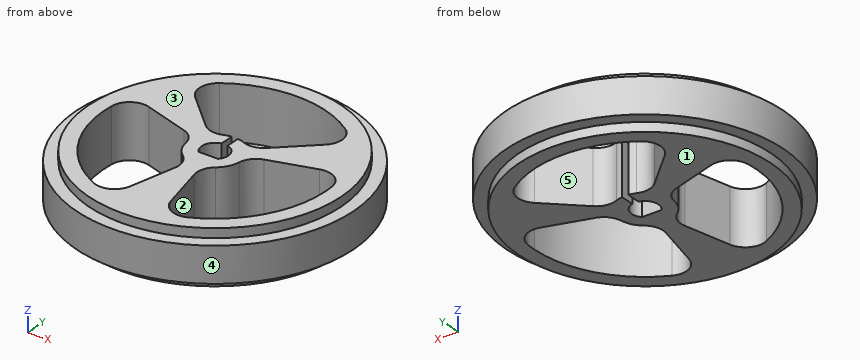
```python
from build123d import *

# Parameters (mm, degrees)
F3_DEPTH = 7
F4_R     = 2.5


with BuildPart() as f1:
    # F0 (on Front) → F1 (revolve)
    with BuildSketch(Plane.XZ):
        Polygon((-16.4, 0), (0, 0), (0, 7), (-16.4, 7), (-16.4, 5.8), (-18, 5.8), (-18, 1.2), (-16.4, 1.2), align=None)
    revolve(axis=Axis((0, 0, 3.5), (0, 0, -1)))

    # F2 (on Top) → F3 (cut, through all)
    with BuildSketch(Plane.XY):
        with BuildLine():
            Line((-0.4, 3.477068), (-0.4, 1.677982))
            ThreePointArc((-0.4, 1.677982), (-1.651125, 0.499411), (-1.262933, -1.175))
            Line((-1.262933, -1.175), (1.262933, -1.175))
            ThreePointArc((1.262933, -1.175), (1.651125, 0.499411), (0.4, 1.677982))
            Line((0.4, 1.677982), (0.4, 3.477068))
            ThreePointArc((0.4, 3.477068), (1.573642, 3.126284), (2.55453, 2.392567))
            Line((2.55453, 2.392567), (10.510067, 9.843703))
            ThreePointArc((10.510067, 9.843703), (0, 14.4), (-10.510067, 9.843703))
            Line((-10.510067, 9.843703), (-2.55453, 2.392567))
            ThreePointArc((-2.55453, 2.392567), (-1.573642, 3.126284), (-0.4, 3.477068))
        make_face()
        with BuildLine():
            ThreePointArc((3.349289, 1.016005), (3.031089, -1.75), (0.794758, -3.408571))
            Line((0.794758, -3.408571), (3.269863, -14.023837))
            ThreePointArc((3.269863, -14.023837), (11.279318, -8.951926), (14.4, 0))
            ThreePointArc((14.4, 0), (14.244139, 2.112937), (13.77993, 4.180134))
            Line((13.77993, 4.180134), (3.349289, 1.016005))
        make_face()
        with BuildLine():
            ThreePointArc((-0.794758, -3.408571), (-3.031089, -1.75), (-3.349289, 1.016005))
            Line((-3.349289, 1.016005), (-13.77993, 4.180134))
            ThreePointArc((-13.77993, 4.180134), (-12.470766, -7.2), (-3.269863, -14.023837))
            Line((-3.269863, -14.023837), (-0.794758, -3.408571))
        make_face()
    extrude(amount=F3_DEPTH, mode=Mode.SUBTRACT)

    # F4
    f4_edges = [f1.edges().sort_by_distance(p)[0] for p in [
        (-3.349289, 1.016005, 3.5),
        (-0.794758, -3.408571, 3.5),
        (0.794758, -3.408571, 3.5),
        (3.349289, 1.016005, 3.5),
        (-2.55453, 2.392567, 3.5),
        (2.55453, 2.392567, 3.5),
        (-10.510067, 9.843703, 3.5),
        (10.510067, 9.843703, 3.5),
        (13.77993, 4.180134, 3.5),
        (3.269863, -14.023837, 3.5),
        (-3.269863, -14.023837, 3.5),
        (-13.77993, 4.180134, 3.5),
    ]]
    fillet(f4_edges, radius=F4_R)


solid = f1.part
```
The model under review builds one solid part; all positions refer to its coordinate system, in mm. Face numbers are marked on the shaded views. A direction names the side the tool comes from. Give positions to 0.01 mm unless a question says otherwise; leave off trailing zeros. Write each loop counter-clockwise with the first axis right and the second up, starting at its lowest first coordinate (ties: lowest second). Pieces come first, ordered by that corner, then holes. Notation, with made-up numbers: M 44.5,55.25 L 85.5,55.25 A20 cw 85.5,74.25 Z; hole C -1.75,-39.5 d2. An arc over 180 degrees is marked long. Write item = value, one per line. Start each with the question number.
Q1. We need section D-D (y = 10). State the section outline as (x, z) points, plus the area to 3 significant figures.
Q2. We need section C-C (x = -13.5). State the section outline as (y, z) points, plus the area to 3 significant figures.
Q3. For line 1 (Y direction, x = 8, z = 5.5); line 2 (Y direction, x = 8.5, z = 6.25); line 3 (X direction, y = -4.5, z = 6), list the stretches that pass through material, from the lowest coordinate up.
Q4. Clearance check with flat-ended pins moving along their axes: pin 1 (1.4 mm diameter, centred on y = 2.5, z = 4.5, fed in from +X); pin 2 (2 mm diameter, centred on y = 2.5, z = 4.5, fed in from -X); pin 3 (1.5 mm diameter, centred on y = 9.5, z = 1, fed in from +X) (3 decimals). State where each tip first meets the part, or that it passes through.
Q5. Machinability: for the marked faces 1 and 2, which of the approach directions +Z, -Z, +X, -X, +Y, -Y give a long, thin tool a straight path to every point of the face, cutting with its end or side? Answer none if there is none.
Q6. Mouldability with a two-part tool opening along X and no side actions: class the marked faces 3, 4 and 5 as released by +X, released by -X, zero draft, split by the parting line, or undercut.
Q7. We need section A-A (z = 4.25). Give the number of separate pieces and of enclosed holes in the cut face, plus the area to 3 significant figures.
Q8. We need section B-B (y = -7). State the section outline as (x, z) points, plus the area to 3 significant figures.
Result set:
q1.outline = M -14.97,1.2 L -13,1.2 L -13,0 L -9.27,0 L -9.27,7 L -13,7 L -13,5.8 L -14.97,5.8 Z; M 9.27,0 L 13,0 L 13,1.2 L 14.97,1.2 L 14.97,5.8 L 13,5.8 L 13,7 L 9.27,7 Z
q1.area = 70.3 mm2
q2.outline = M -11.91,1.2 L -9.31,1.2 L -9.31,0 L -5.01,0 L -5.01,7 L -9.31,7 L -9.31,5.8 L -11.91,5.8 Z; M 2.87,0 L 9.31,0 L 9.31,1.2 L 11.91,1.2 L 11.91,5.8 L 9.31,5.8 L 9.31,7 L 2.87,7 Z
q2.area = 99.1 mm2
q3.line_1 = -16.12 to -11.97, 2.43 to 7.49, 11.97 to 16.12
q3.line_2 = -14.03 to -11.62, 2.58 to 7.96, 11.59 to 14.03
q3.line_3 = -15.77 to -13.68, -1.19 to 1.19, 13.68 to 15.77
q4.pin_1 = 17.91
q4.pin_2 = -17.94
q4.pin_3 = 15.715
q5.face_1 = -Z, +X, -X, +Y, -Y
q5.face_2 = +Z, -Z
q6.face_3 = zero draft
q6.face_4 = split by the parting line
q6.face_5 = undercut
q7.separate_pieces = 1
q7.enclosed_holes = 3
q7.area = 544 mm2
q8.outline = M -16.58,1.2 L -14.83,1.2 L -14.83,0 L -12.58,0 L -12.58,7 L -14.83,7 L -14.83,5.8 L -16.58,5.8 Z; M -1.63,0 L 1.63,0 L 1.63,7 L -1.63,7 Z; M 12.58,0 L 14.83,0 L 14.83,1.2 L 16.58,1.2 L 16.58,5.8 L 14.83,5.8 L 14.83,7 L 12.58,7 Z
q8.area = 70.4 mm2
